Read the model definition and answer for the solid it produces. Units are mm, in the model's axes. Round coordinates to 2 decimals unless told otherwise and drop trailing zeros. Write each loop counter-clockwise with the first axis right and the second up, starting at its lowest first coordinate (ties: lowest second). Pieces come first, ordered by that corner, then holes. Notation, with made-up numbers: M 34.25,-21 L 47.25,-21 A31 cw 47.25,7 Z; hole C 48.5,10.5 d10. An arc over 180 degrees is marked long. Use one line per item in the form item = value. Start each with the question number.
Autodesk Inventor part; units mm, degrees
ref_plane "Work Plane2" through (1.5, 0, 0) normal (1, 0, 0) x (0, 0, -1)
ref_plane "YZ Plane" through (0, 0, 0) normal (1, 0, 0) x (0, 1, 0)
ref_plane "XZ Plane" through (0, 0, 0) normal (0, 1, 0) x (-1, 0, 0)
sketch "Sketch1" plane through (0, 0, 0) normal (1, 0, 0) x (0, 1, 0)
  circle A0 centre (0, 0) radius 2.05
  dimension "d0" = 4.1
extrude "Extrusion1" add sketch "Sketch1" against normal blind 38
ref_plane "Work Plane1" through (1, 0, 0) normal (1, 0, 0) x (0, 0, -1)
sketch "Sketch2" plane through (1, 0, 0) normal (1, 0, 0) x (0, 0, -1)
  circle A0 centre (0, 0) radius 3
  dimension "d4" = 6
loft "Loft1" add profiles "Sketch2" section 1 edges at (0, -2.05, 0)
sketch "Sketch3" plane through (0, 0, 0) normal (0, 1, 0) x (-1, 0, 0)
  line L0 (-1, -3) -> (-1, 3)
  line L1 (-1, 3) -> (-1, 0)
  line L2 (-1, 0) -> (-1.5, 0)
  arc A0 (-1, 3) -> (-1.5, 0) centre (7.75, 0) ccw
  point P0 (0, 0)
  dimension "d9" = 0.5
revolve "Revolution1" add sketch "Sketch3" angle 360 about axis through (1, 0, 0) along (1, 0, 0)
ref_plane "Work Plane2" through (1.5, 0, 0) normal (1, 0, 0) x (0, 0, -1)
sketch "Sketch4" plane through (1.5, 0, 0) normal (1, 0, 0) x (0, 0, -1)
  line L0 (2, 0.5) -> (2, -0.5)
  line L1 (-2, -0.5) -> (-2, 0.5)
  line L2 (-0.5, 2) -> (0.5, 2)
  line L3 (0.5, -2) -> (-0.5, -2)
  line L4 (2, -0.5) -> (0.5, -0.5)
  line L5 (-0.5, -0.5) -> (-2, -0.5)
  line L6 (-0.5, -2) -> (-0.5, -0.5)
  line L7 (-0.5, 0.5) -> (-0.5, 2)
  line L8 (-2, 0.5) -> (-0.5, 0.5)
  line L9 (0.5, 0.5) -> (2, 0.5)
  line L10 (0.5, 2) -> (0.5, 0.5)
  line L11 (0.5, -0.5) -> (0.5, -2)
  dimension "d12" = 4
  dimension "d13" = 1
  dimension "d14" = 1
  dimension "d15" = 4
extrude "Extrusion2" cut sketch "Sketch4" against normal blind 1 draft -10
chamfer "Chamfer1" distance 0.5 angle 45 1 edges at (-38, -2.05, 0)
thread "Thread1"
properties part number "Parafuso do Braço (2)"
Q1. Each of these flat-tipped pins is pushed along its axis until it touches: pin 1 Ø2 at (x, y) = (-10, 1) entering from -Z; pin 2 Ø1.5 at (y, z) = (-1, 1.5) entering from +X. Where does it stop, or does it pass through?
Q2. Straight lines are drawn through the part: line 1 (X direction, y = 0.25, z = 1.25); line 2 (X direction, y = 2.5, z = -0.5); line 3 (Z direction, x = -17, y = -0.75). For each, find the intervals that lie inside material, in ascending order. Write a range as [from, to].
Q3. For a pull along Z with two mould halves and no side action, classify faces 1 (the face through (-38, 0, 0)), 2 (the face through (0.99, -0.41, -1.15)), 3 (the face through (-18.488, -0.267, 2.033)) as +Z half, -Z half, draft (parallel to the pull), parting line (faces both ways), or undercut.
Q4. Find section A-A on y = 0. Write down the section's boundary in (x, z).
Q5. Find section B-B on x = -2. Write down the section's boundary in (y, z).
Response:
q1.pin_1 = -2.05
q1.pin_2 = 1.44
q2.line_1 = [-38, 0.5]
q2.line_2 = [0.53, 1.14]
q2.line_3 = [-1.91, 1.91]
q3.face_1 = draft
q3.face_2 = undercut
q3.face_3 = parting line
q4.outline = M -38,-1.55 L -37.5,-2.05 L 0,-2.05 L 1,-3 A9.25 ccw 1.29,-1.96 L 0.5,-1.82 L 0.5,1.82 L 1.29,1.96 A9.25 ccw 1,3 L 0,2.05 L -37.5,2.05 L -38,1.55 Z
q5.outline = C 0,0 d4.1
